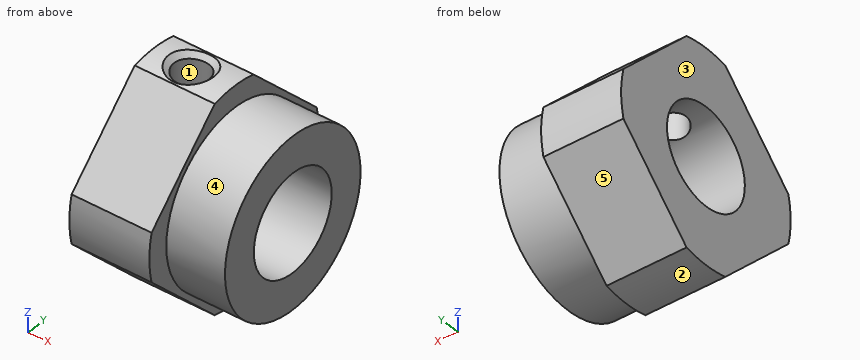
Autodesk Inventor part; units mm, degrees
ref_plane "YZ Plane" through (0, 0, 0) normal (1, 0, 0) x (0, 1, 0)
ref_plane "XZ Plane" through (0, 0, 0) normal (0, 1, 0) x (-1, 0, 0)
ref_plane "XY Plane" through (0, 0, 0) normal (0, 0, 1) x (1, 0, 0)
sketch "Sketch1" plane through (0, 0, 0) normal (0, 0, 1) x (1, 0, 0)
  line L0 (0, 10) -> (0, 0)
  line L1 (0, 10) -> (7.5, 10)
  line L2 (7.5, 10) -> (7.5, 8)
  line L3 (7.5, 8) -> (13, 8)
  line L4 (13, 8) -> (13, 0)
  line L5 (13, 0) -> (0, 0)
  point P0 (0, 0)
  dimension "d0" = 16
  dimension "d1" = 20
  dimension "d2" = 13
  dimension "d3" = 7.5
revolve "Revolution1" add sketch "Sketch1" angle 360 about axis through (13, 0, 0) along (-1, 0, 0)
hole "Hole1" at (0, 0, 0) direction (1, 0, 0) diameter 9.188 end through all
sketch "Sketch2" plane through (0, 0, 0) normal (-1, 0, 0) x (0, 0, 1)
  line L0 (0, -12.0208) -> (12.0208, 0)
  line L1 (12.0208, 0) -> (0, 12.0208)
  line L2 (0, 12.0208) -> (-12.0208, 0)
  line L3 (-12.0208, 0) -> (0, -12.0208)
  line L4 (0, -12.0208) -> (0, 12.0208) construction
  line L5 (12.0208, 0) -> (-12.0208, 0) construction
  line L6 (0, -11.9) -> (0, 11.9)
  point P0 (0, 0)
  dimension "d14" = 17
extrude "Extrusion1" cut sketch "Sketch2" against normal through all keep common part
sketch "Sketch3" plane through (0, 0, 0) normal (0, 0, 1) x (1, 0, 0)
  line L0 (0, -2.2855) -> (0, 2.2855)
  point P0 (0, 0)
  point P1 (3.5, 0)
  point P2 (0, 0)
  dimension "d17" = 3.5
hole "Hole2" at (3.5, 0, 0) direction (0, 0, 1) diameter 3.242 end through all
chamfer "Chamfer1" distance 0.5 angle 45 1 edges at (3.4896, -1.621, 9.8677)
properties part number "Wellenmutter" material "Steel"
The model under review builds one solid part; all positions refer to its coordinate system, in mm. Face numbers are marked on the shaded views. A direction names the side the tool comes from. Coordinates: 2 decimals unless noted, no trailing zeros. Loops run counter-clockwise (first coordinate to the right, second up) from the corner with the lowest first, then second, coordinate; pieces in that order, holes last. Notation, with made-up numbers: M -27,-22.75 L -13,-22.75 A23 cw -13,12.25 Z; hole C 78,65.5 d7. An arc over 180 degrees is marked long. Put each result on its own line as item: value. Start each with the question number.
Q1. Clearance check with flat-ended pins moving along their axes: pin 1 (3.5 mm diameter, centred on x = 3.5, y = 0, fed in from +Z); pin 2 (5 mm diameter, centred on x = 2.5, y = 8, fed in from +Z). State where each tip first meets the part, or that it passes through.
Q2. The part is to be moulded in two halves that separate along X. For the marked faces 1, 2 and 3, say which applies: +X half, -X half, draft (parallel to the pull), parting line (faces both ways), or undercut.
Q3. Wall thickness on line 1 (X direction, y = 0, z = 5.4); line 2 (Z direction, x = 10.5, y = 0); line 3 (Z direction, x = 4.5, y = -2.25): over which ranges is each line inside the solid? List them lowest first.
Q4. Add section D-D (z = -5). Write out the cut boundary in (x, y) (3 decimals).
Q5. Add section C-C (x = 8.5). Write out the cut boundary in (y, z).
Q6. Add section A-A (y = 4). Write out the cut boundary in (x, z).
Q7. Add section B-B (z = -1). Write out the cut boundary in (x, y).
Q8. For the marked faces 4 and 5, list the 3-axis set-ups (+Z, -Z, +X, -X, +Y, -Y) from which the entire face can be reached by the end or side of a thin tool; tool diameter is ignored.
Answers:
1. pin 1: stops at z = 9.63
1. pin 2: stops at z = 6.52
2. face 1: undercut
2. face 2: draft
2. face 3: -X half
3. line 1: x = 0 to 1.88, 5.12 to 13
3. line 2: z = -8 to -4.59, 4.59 to 8
3. line 3: z = -9.74 to -4.01, 4.01 to 9.74
4. outline: M 0,-7.021 L 7.5,-7.021 L 7.5,-6.245 L 13,-6.245 L 13,6.245 L 7.5,6.245 L 7.5,7.021 L 0,7.021 Z
5. outline: C 0,0 d16; hole C 0,0 d9.19
6. outline: M 0,-8.02 L 7.5,-8.02 L 7.5,-6.93 L 13,-6.93 L 13,-2.26 L 0,-2.26 Z; M 0,2.26 L 13,2.26 L 13,6.93 L 7.5,6.93 L 7.5,8.02 L 0,8.02 Z
7. outline: M 0,-9.95 L 7.5,-9.95 L 7.5,-7.94 L 13,-7.94 L 13,-4.48 L 0,-4.48 Z; M 0,4.48 L 13,4.48 L 13,7.94 L 7.5,7.94 L 7.5,9.95 L 0,9.95 Z
8. face 4: +X
8. face 5: -Z, +X, -X, +Y
